Here's how the part is built. I have some questions about the finished solid (model axes, mm). Face numbers are marked on the shaded views. A direction names the side the tool comes from. Give positions to 0.01 mm unless a question says otherwise; leave off trailing zeros. Loops run counter-clockwise (first coordinate to the right, second up) from the corner with the lowest first, then second, coordinate; pieces in that order, holes last. Notation, with made-up numbers: M 70,71.25 L 111,71.25 A20 cw 111,95.25 Z; hole C 71.25,8.5 d9. An arc over 180 degrees is marked long. Answer as CSV lines item,"result". Start each with the question number.
Item 1: I want a section at A-A on z = 0. Give the number of separate pieces and of enclosed holes in the cut face, plus the area to 3 significant figures.
Item 2: If we mould it in two halves opening along Z, with no side actions, what happens to the marked faces 1, 2 and 3? For each: released by +Z, released by -Z, zero draft, split by the parting line, or undercut.
Item 3: For the marked faces 4 and 5, which set-ups out of +Z, -Z, +X, -X, +Y, -Y let a thin tool reach every point of the face, with its end or its side?
Item 4: If I drill on line 1 along X through (y, z) = (10.5, -8.25); line 2 along Z through (x, y) = (2.75, 13), over which ranges is the centre line in solid material (lowest first)? Write a range as from..to.
Item 5: I want a section at C-C on y = 11.5. List the corners of the cut face in (x, z) for me, plus the area to 3 significant figures.
Item 6: I want a section at B-B on x = 13.5. List the corners of the cut face in (y, z) for me, plus the area to 3 significant figures.
Item 7: Will these pins go through, and if not, where does the flat tip stop? P1, Ø1.5, axis at x = 13.5, z = 1.5, coming from the +Y side; P2, Ø1.5, axis at y = 6, z = 4, coming from the +X side; P3, Ø11, axis at y = 15.5, z = -5.5, coming from the +X side; P4, Ø6, axis at x = 17, z = 5, coming from the +Y side.
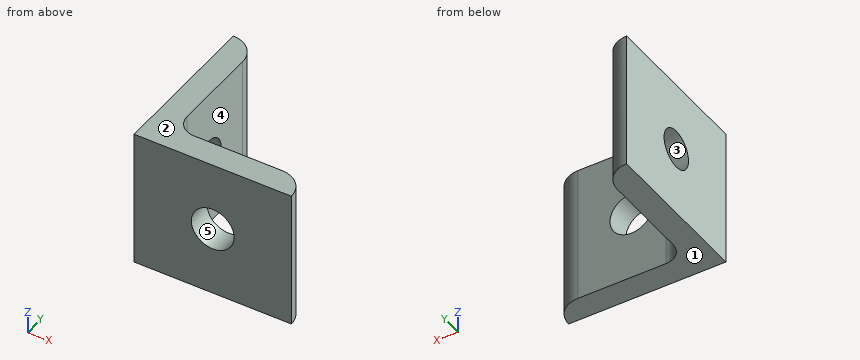
from build123d import *

# Parameters (mm, degrees)
BOSS_EXTRUDE1_DEPTH = 10.9982
FILLET1_R           = 4
FILLET2_R           = 3
CUT_EXTRUDE1_REACH  = 39.026
SKETCH2_R           = 3.4036
CUT_EXTRUDE2_REACH  = 39.026
SKETCH4_R           = 3.075953135


with BuildPart() as part:
    # Sketch1 → Boss-Extrude1 (new, symmetric)
    with BuildSketch(Plane.XY):
        Polygon((0, 0), (0, 25), (4, 25), (4, 4), (25, 4), (25, 0), align=None)
    extrude(amount=BOSS_EXTRUDE1_DEPTH, both=True)

    # Fillet1
    fillet1_edges = [part.edges().sort_by_distance(p)[0] for p in [
        (25, 4, 0),
        (4, 25, 0),
    ]]
    fillet(fillet1_edges, radius=FILLET1_R - 0.0001)  # a hair under: the kernel refuses the full size

    # Fillet2
    fillet2_edges = [part.edges().sort_by_distance(p)[0] for p in [
        (4, 4, 0),
    ]]
    fillet(fillet2_edges, radius=FILLET2_R)

    # Sketch2 → Cut-Extrude1 (cut, up to next)
    with BuildSketch(Plane.XZ, mode=Mode.PRIVATE) as cut_extrude1_sk1:
        with Locations((12.4968, 0)):
            Circle(SKETCH2_R)
    cut_extrude1_tool1 = extrude(cut_extrude1_sk1.sketch, amount=-CUT_EXTRUDE1_REACH, mode=Mode.PRIVATE) & part.part
    add(cut_extrude1_tool1.solids().sort_by_distance((12.4968, 0, 0))[0], mode=Mode.SUBTRACT)

    # Sketch4 → Cut-Extrude2 (cut, up to next)
    with BuildSketch(Plane.ZY, mode=Mode.PRIVATE) as cut_extrude2_sk1:
        with Locations((0, 12.4968)):
            Circle(SKETCH4_R)
    cut_extrude2_tool1 = extrude(cut_extrude2_sk1.sketch, amount=-CUT_EXTRUDE2_REACH, mode=Mode.PRIVATE) & part.part
    add(cut_extrude2_tool1.solids().sort_by_distance((0, 12.4968, 0))[0], mode=Mode.SUBTRACT)


solid = part.part
Result:
1,separate pieces,"3"
1,enclosed holes,"0"
1,area,"127 mm^2"
2,face 1,"released by -Z"
2,face 2,"released by +Z"
2,face 3,"undercut"
3,face 4,"+Z, -Z, +X, +Y"
3,face 5,"+Y, -Y"
4,line 1,"0..4"
4,line 2,"-11..-3.03, 3.03..11"
5,outline,"M 0,-11 L 4,-11 L 4,-2.91 L 0,-2.91 Z; M 0,2.91 L 4,2.91 L 4,11 L 0,11 Z"
5,area,"64.7 mm^2"
6,outline,"M 0,-11 L 4,-11 L 4,-3.25 L 0,-3.25 Z; M 0,3.25 L 4,3.25 L 4,11 L 0,11 Z"
6,area,"62.0 mm^2"
7,P1,"through"
7,P2,"x = 4.56"
7,P3,"x = 4"
7,P4,"y = 4"
